Model file for the job. Use its own axes, mm. Give positions to 0.01 mm unless a question says otherwise; leave off trailing zeros. Loops run counter-clockwise (first coordinate to the right, second up) from the corner with the lowest first, then second, coordinate; pieces in that order, holes last. Notation, with made-up numbers: (58.5, 64) - (104.5, 64) arc R22 ccw to (104.5, 77) - close; hole circle Ø10 at (-36.75, -22). An arc over 180 degrees is marked (long way). Use a Markdown table: item, result.
Autodesk Inventor part; units mm, degrees
ref_plane "Work Plane2" through (-135.0962, 102.1952, 0) normal (-0.9486, -0.3165, 0) x (0.3165, -0.9486, 0)
ref_plane "YZ Plane" through (0, 0, 0) normal (1, 0, 0) x (0, 1, 0)
ref_plane "XZ Plane" through (0, 0, 0) normal (0, 1, 0) x (-1, 0, 0)
sketch "Sketch1" plane through (0, 0, 0) normal (0, 0, 1) x (1, 0, 0)
  line L0 (0, 0) -> (3321.2151, 1108.1486)
  line L1 (3321.2151, 1255.4197) -> (-135.0962, 102.1952)
  line L2 (0, 0) -> (-135.0962, 0)
  line L3 (-135.0962, 0) -> (-135.0962, 102.1952)
  line L4 (-135.0962, 102.1952) -> (1593.1098, 678.8242)
  line L5 (3321.2151, 1108.1486) -> (3263.9, 1108.1486)
  line L6 (3321.2151, 1108.1486) -> (3321.2151, 1255.4197)
  line L7 (-88.9, 0) -> (-88.9, 117.6089)
  line L8 (3263.9, 1089.025) -> (3263.9, 1236.2961)
  line L9 (-135.0962, 102.1952) -> (-135.0962, 118.9305)
  line L10 (-135.0962, 118.9305) -> (1016.4014, 503.1364)
  line L11 (1016.4014, 503.1364) -> (1021.4259, 488.0776)
  line L12 (1021.4259, 488.0776) -> (-135.0962, 102.1952)
  line L13 (-135.0962, 102.1952) -> (-100.9981, 0)
  line L14 (3321.2151, 1255.4197) -> (3321.2151, 1272.155)
  line L15 (3321.2151, 1272.155) -> (2171.3189, 888.4834)
  line L16 (2171.3189, 888.4834) -> (2176.3434, 873.4245)
  dimension "d5" = 139.7
  dimension "d17" = 88.9
  dimension "d19" = 3352.8
  dimension "d23" = 57.3151
  dimension "d28" = 46.1962
  dimension "d33" = 1089.025
  dimension "d36" = 15.875
  dimension "d37" = 1219.2
  dimension "d41" = 15.875
  dimension "d42" = 1212.215
extrude "Extrusion2" add sketch "Sketch1" along normal blind 2438.4 contours L1 L16 L15 L14
ref_plane "Work Plane2" through (-135.0962, 102.1952, 0) normal (-0.9486, -0.3165, 0) x (0.3165, -0.9486, 0)
properties part number "OSB_For_Front_Roof" material "Wood (Birch)"
(1) Slice it at C-C, the plane y = 1032.5. Write the cut outline in (x, z).
Computed:
| item | result |
|---|---|
| outline | (2602.95, 0) - (2653.11, 0) - (2653.11, 2438.4) - (2602.95, 2438.4) - close |
(2) Drill centre lines: probe 1 along Y at (x, z) = (2792, 1914.5); probe 2 along Y at (x, z) = (2806, 1533.5). Where is each one in solid material? Low to high. Write a range as [from, to].
Computed:
| item | result |
|---|---|
| probe 1 | [1078.84, 1095.58] |
| probe 2 | [1083.51, 1100.25] |
(3) Slice it at A-A, the plane z = 1690.5. Write the cut outline in (x, y) (1 decimal), plus the area to 3 significant figures.
Computed:
| item | result |
|---|---|
| outline | (2171.3, 888.5) - (2176.3, 873.4) - (3321.2, 1255.4) - (3321.2, 1272.2) - close |
| area | 19,200 mm² |
(4) Pin check, flat tips, straight feed: P1, Ø10, axis at x = 2647, z = 1006, coming from the +Y side; P2, Ø3, axis at x = 3104.5, z = 2054.5, coming from the -Y side; P3, Ø12, axis at x = 2634, z = 703.5, coming from the -Y side. Stop position of each tip, or through.
Computed:
| item | result |
|---|---|
| P1 | y = 1048.87 |
| P2 | y = 1182.61 |
| P3 | y = 1024.12 |
(5) Slice it at B-B, the plane x = 3226.5. Write the cut outline in (y, z).
Computed:
| item | result |
|---|---|
| outline | (1223.82, 0) - (1240.55, 0) - (1240.55, 2438.4) - (1223.82, 2438.4) - close |
